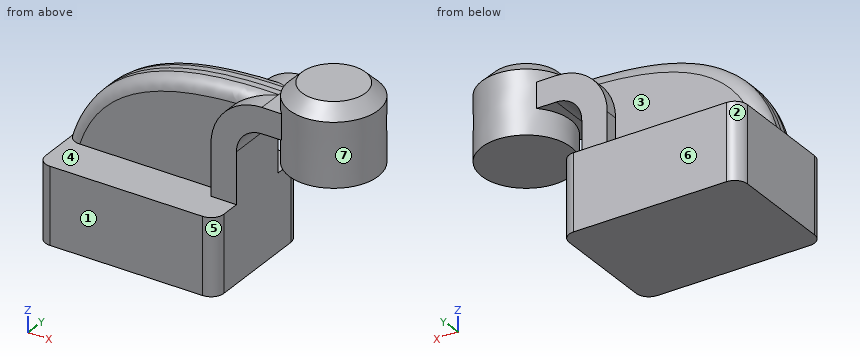
```python
from build123d import *

# Parameters (mm, degrees)
F1_DEPTH = 25
F2_DEPTH = 7.5
F3_DEPTH = 12.5
F4_DEPTH = 12.5
F6_R     = 5
F7_SIZE  = 5


with BuildPart() as f1:
    # F0 (on Front) → F1 (new body, symmetric)
    with BuildSketch(Plane.XZ):
        Polygon((25, 15), (-35, 15), (-35, -15), (35, -15), (35, 15), align=None)
    extrude(amount=F1_DEPTH, both=True)

    # F0 (on Front) → F2 (join, symmetric)
    with BuildSketch(Plane.XZ):
        with BuildLine():
            add(Edge.make_bspline(
                [(-35, 15), (-25.293957442, 48.5758967698), (8.6229406297, 55.761680007), (45, 55)],
                knots=[0, 0, 0, 0, 89.4427191, 89.4427191, 89.4427191, 89.4427191], degree=3))
            Line((-35, 15), (25, 15))
            Line((25, 15), (25, 35))
            ThreePointArc((25, 35), (30.8578643763, 49.1421356237), (45, 55))
        make_face()
    extrude(amount=F2_DEPTH, both=True)

    # F0 (on Front) → F3 (join, symmetric)
    with BuildSketch(Plane.XZ):
        with BuildLine():
            Line((25, 35), (25, 15))
            Line((25, 15), (35, 15))
            Line((35, 15), (35, 35))
            ThreePointArc((35, 35), (37.9289321881, 42.0710678119), (45, 45))
            Line((45, 45), (47.4594813585, 45))
            Line((47.4594813585, 45), (47.4594813585, 55))
            Line((47.4594813585, 55), (45, 55))
            ThreePointArc((45, 55), (30.8578643763, 49.1421356237), (25, 35))
        make_face()
    extrude(amount=F3_DEPTH, both=True)

    # F0 (on Front) → F4 (join, symmetric)
    with BuildSketch(Plane.XZ):
        Polygon((64.9868643671, 55), (47.4594813585, 55), (47.4594813585, 45), (64.9733581532, 45), align=None)
    extrude(amount=F4_DEPTH, both=True)

    # F0 (on Front) → F5 (revolve)
    with BuildSketch(Plane.XZ):
        Polygon((65, 64.7256219387), (64.9868643671, 55), (64.9733581532, 45), (64.9594813585, 34.7256219387), (82.4594813585, 34.7256219387), (82.4594813585, 64.7256219387), align=None)
    revolve(axis=Axis((64.9797406793, 0, 49.7256219387), (0.0013506202, 0, 0.9999990879)))

    # F6
    f6_edges = [f1.edges().sort_by_distance(p)[0] for p in [
        (35, -25, 0),
        (-35, -25, 0),
        (-35, 25, 0),
        (35, 25, 0),
        (-2.822986, -7.5, 48.736199),
        (-2.822986, 7.5, 48.736199),
    ]]
    fillet(f6_edges, radius=F6_R)

    # F7
    f7_edges = [f1.edges().sort_by_distance(p)[0] for p in [
        (47.540582, 0, 64.772784),
    ]]
    chamfer(f7_edges, length=F7_SIZE)


solid = f1.part
```
Build history of the part. All positions in model axes, mm. Face numbers are marked on the shaded views. A direction names the side the tool comes from. Coordinates: 2 decimals unless noted, no trailing zeros. Order: outer loops, then holes, each group sorted by start corner. A loop starts at its lowest first (then second) coordinate and runs counter-clockwise, first axis right, second up. Notation, with made-up numbers: (61.25, 44.25) -> (76.25, 44.25) arc R18 cw to (76.25, 55.25) -> close; hole circle Ø3 at (-20.75, 12). An arc over 180 degrees is marked (long way). Answer in a Markdown table with one row per item. Add a question column.
Q1. Drop flat-ended pins along their axis: pin 1 (6 mm diameter, centred on x = 33.5, z = 3.5, fed in from +Y); pin 2 (3 mm diameter, centred on x = 0.5, z = 29.5, fed in from +Y); pin 3 (5.5 mm diameter, centred on y = -10.5, z = 22, fed in from -X). Give the stop position or say it passes through.
Q2. Band-saw the part on A-A, the plane z = 9. List the corners of the cut face in (x, y), then the cut area to 3 significant figures.
Q3. Which spindle directions (+Z, -Z, +X, -X, +Y, -Y) get a long thin tool onto all of the face, cutting with end or side? Do the marked faces 1, 2, 3 and 4. Say none if no direction does.
Q4. Mould opens along X. For the marked faces 5, 6 and 7 say: +X half, -X half, draft (parallel to the pull), parting line (faces both ways), or undercut.
Q5. Wall check: line 1 along X through (y, z) = (3, 8); line 2 along Z through (x, y) = (30, 17); line 3 along Z through (x, y) = (65, 8.5). Give the ranges that are in metal, low to high. Write a range as [from, to].
Answers follow:
| question | item | result |
|---|---|---|
| 1 | pin 1 | y = 24.97 |
| 1 | pin 2 | y = 7.5 |
| 1 | pin 3 | x = 25 |
| 2 | outline | (-35, -20) arc R5 ccw to (-30, -25) -> (30, -25) arc R5 ccw to (35, -20) -> (35, 20) arc R5 ccw to (30, 25) -> (-30, 25) arc R5 ccw to (-35, 20) -> close |
| 2 | area | 3,480 mm^2 |
| 3 | face 1 | +Z, -Z, +X, -X, -Y |
| 3 | face 2 | +Z, -Z, -X, +Y |
| 3 | face 3 | +Z, -X, +Y |
| 3 | face 4 | +Z, -X, -Y |
| 4 | face 5 | +X half |
| 4 | face 6 | draft |
| 4 | face 7 | undercut |
| 5 | line 1 | [-35, 35] |
| 5 | line 2 | [-15, 15] |
| 5 | line 3 | [34.74, 64.74] |
